Autodesk Inventor part; units mm, degrees
ref_plane "YZ Plane" through (0, 0, 0) normal (1, 0, 0) x (0, 1, 0)
ref_plane "XZ Plane" through (0, 0, 0) normal (0, 1, 0) x (-1, 0, 0)
ref_plane "XY Plane" through (0, 0, 0) normal (0, 0, 1) x (1, 0, 0)
sketch "Sketch1" plane through (0, 0, 0) normal (0, 0, 1) x (1, 0, 0)
  circle A0 centre (0, 4) radius 2 construction
  circle A1 centre (-195, 4) radius 2 construction
  circle A2 centre (195, 4) radius 2 construction
  arc A3 (213, -12) -> (215, -10) centre (213, -10) ccw construction
  line L0 (215, -10) -> (215, 10) construction
  arc A4 (215, 10) -> (213, 12) centre (213, 10) ccw construction
  line L1 (213, 12) -> (-213, 12) construction
  line L2 (94, -2.8) -> (94, -7.2) construction
  line L3 (94, -7.2) -> (87.6, -7.2) construction
  line L4 (87.6, -7.2) -> (87.6, -2.8) construction
  line L5 (87.6, -2.8) -> (94, -2.8) construction
  line L6 (-108.8, -2.8) -> (-108.8, -7.2) construction
  line L7 (-108.8, -7.2) -> (-115.2, -7.2) construction
  line L8 (-115.2, -7.2) -> (-115.2, -2.8) construction
  line L9 (-115.2, -2.8) -> (-108.8, -2.8) construction
  line L10 (115.2, -2.8) -> (115.2, -7.2) construction
  line L11 (115.2, -7.2) -> (108.8, -7.2) construction
  line L12 (108.8, -7.2) -> (108.8, -2.8) construction
  line L13 (108.8, -2.8) -> (115.2, -2.8) construction
  line L14 (-87.6, -2.8) -> (-87.6, -7.2) construction
  line L15 (-87.6, -7.2) -> (-94, -7.2) construction
  line L16 (-94, -7.2) -> (-94, -2.8) construction
  line L17 (-94, -2.8) -> (-87.6, -2.8) construction
  circle A5 centre (-101.4, -5) radius 1.6 construction
  circle A6 centre (101.4, -5) radius 1.6 construction
  line L18 (213.9083, -46) -> (-214.0917, -46) construction
  line L19 (-225, 12) -> (225, 12)
  line L20 (225, 12) -> (225, -46)
  line L21 (-225, -46) -> (-225, 12)
  line L22 (-225, -46) -> (225, -46)
  line L23 (197, -54.5741) -> (193, -54.5741)
  line L24 (2, -54.5741) -> (-2, -54.5741)
  line L25 (-195, -54.5741) -> (-197, -54.5741)
  line L26 (-108.8, -54.5741) -> (-115.2, -54.5741)
  line L27 (94, -54.5741) -> (87.6, -54.5741)
  line L28 (-225, -46) -> (225, -46)
  line L29 (225, -46) -> (225, -48)
  line L30 (225, -48) -> (-225, -48)
  line L31 (-225, -48) -> (-225, -46)
  line L32 (-195, 4) -> (-195, 0) construction
  line L33 (-197, 4) -> (-197, 0)
  line L34 (-193, 0) -> (-193, 4)
  arc A7 (-193, 4) -> (-197, 4) centre (-195, 4) ccw
  arc A8 (-197, 0) -> (-193, 0) centre (-195, 0) ccw
  line L35 (0, 4) -> (0, 0) construction
  line L36 (-2, 4) -> (-2, 0)
  line L37 (2, 0) -> (2, 4)
  arc A9 (2, 4) -> (-2, 4) centre (0, 4) ccw
  arc A10 (-2, 0) -> (2, 0) centre (0, 0) ccw
  line L38 (195, 4) -> (195, 0) construction
  line L39 (193, 4) -> (193, 0)
  line L40 (197, 0) -> (197, 4)
  arc A11 (197, 4) -> (193, 4) centre (195, 4) ccw
  arc A12 (193, 0) -> (197, 0) centre (195, 0) ccw
  circle A13 centre (0, 4) radius 2 construction
  circle A14 centre (-195, 4) radius 2 construction
  circle A15 centre (195, 4) radius 2 construction
  arc A16 (213, -12) -> (215, -10) centre (213, -10) ccw construction
  line L41 (215, -10) -> (215, 10) construction
  arc A17 (215, 10) -> (213, 12) centre (213, 10) ccw construction
  line L42 (213, 12) -> (-213, 12) construction
  arc A18 (-213, 12) -> (-215, 10) centre (-213, 10) ccw construction
  line L43 (-215, 10) -> (-215, -10) construction
  arc A19 (-215, -10) -> (-213, -12) centre (-213, -10) ccw construction
  line L44 (-213, -12) -> (213, -12) construction
  line L45 (94, -2.8) -> (94, -7.2) construction
  line L46 (94, -7.2) -> (87.6, -7.2) construction
  line L47 (87.6, -7.2) -> (87.6, -2.8) construction
  line L48 (87.6, -2.8) -> (94, -2.8) construction
  line L49 (-108.8, -2.8) -> (-108.8, -7.2) construction
  line L50 (-108.8, -7.2) -> (-115.2, -7.2) construction
  line L51 (-115.2, -7.2) -> (-115.2, -2.8) construction
  line L52 (-115.2, -2.8) -> (-108.8, -2.8) construction
  line L53 (115.2, -2.8) -> (115.2, -7.2) construction
  line L54 (115.2, -7.2) -> (108.8, -7.2) construction
  line L55 (108.8, -7.2) -> (108.8, -2.8) construction
  line L56 (108.8, -2.8) -> (115.2, -2.8) construction
  line L57 (-87.6, -2.8) -> (-87.6, -7.2) construction
  line L58 (-87.6, -7.2) -> (-94, -7.2) construction
  line L59 (-94, -7.2) -> (-94, -2.8) construction
  line L60 (-94, -2.8) -> (-87.6, -2.8) construction
  circle A20 centre (-101.4, -5) radius 1.6 construction
  circle A21 centre (101.4, -5) radius 1.6 construction
  point P0 (-213, -12)
  point P1 (-195, 2)
  point P2 (0, 2)
  point P3 (195, 2)
  dimension "d0" = 2
  dimension "d1" = 58
  dimension "d5" = 4
  dimension "d6" = 4
  dimension "d7" = 4
  dimension "d17" = 10
  dimension "d18" = 10
extrude "Extrusion2" add sketch "Sketch1" along normal blind 1
fillet "Fillet2" radius 2 4 edges at (-225, -48, 0.5) (-225, 12, 0.5) (225, 12, 0.5) (225, -48, 0.5)
sketch "Sketch2" plane through (0, 0, 1) normal (0, 0, 1) x (1, 0, 0)
  circle A0 centre (-101.4, -5) radius 1.6
  circle A1 centre (101.4, -5) radius 1.6
  line L0 (115, -3) -> (115, -7)
  line L1 (87.6, -7.2) -> (87.6, -2.8)
  line L2 (-87.8, -3) -> (-87.8, -7)
  line L3 (-115, -3) -> (-115, -7)
  line L4 (-101.4, 24.0788) -> (-101.4, -5) construction
  line L5 (-118.4, 24.0788) -> (-118.4, -5)
  line L6 (-84.4, -5) -> (-84.4, 24.0788)
  arc A2 (-84.4, 24.0788) -> (-118.4, 24.0788) centre (-101.4, 24.0788) ccw
  arc A3 (-118.4, -5) -> (-84.4, -5) centre (-101.4, -5) ccw
  line L7 (101.4, 38.8521) -> (101.4, -5) construction
  line L8 (84.4, 38.8521) -> (84.4, -5)
  line L9 (118.4, -5) -> (118.4, 38.8521)
  arc A4 (118.4, 38.8521) -> (84.4, 38.8521) centre (101.4, 38.8521) ccw
  arc A5 (84.4, -5) -> (118.4, -5) centre (101.4, -5) ccw
  point P0 (-101.4, 9.5394)
  point P1 (101.4, 16.926)
  dimension "d13" = 17
extrude "Extrusion3" cut sketch "Sketch2" against normal blind 1 contours A0 | A1 | A2 L6 A3 L5 | A4 L9 A5 L8
fillet "Fillet3" radius 2 4 edges at (-118.4, 12, 0.5) (-84.4, 12, 0.5) (84.4, 12, 0.5) (118.4, 12, 0.5)
properties part number "wiper 2"
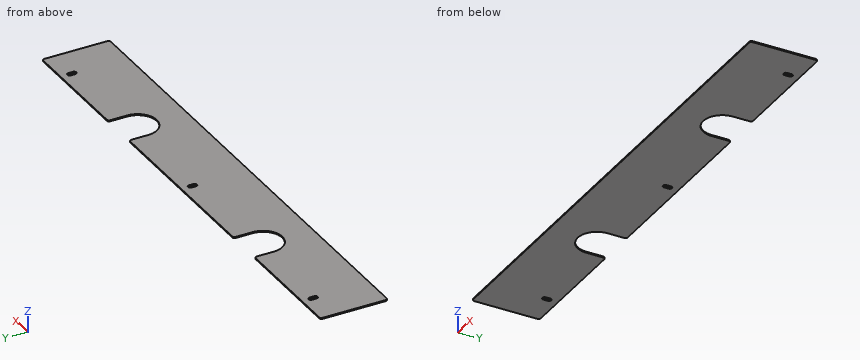
The listing builds one solid part. Answer for the finished solid, in the listing's coordinates (mm). Give positions to 0.01 mm unless a question says otherwise; leave off trailing zeros. Order: outer loops, then holes, each group sorted by start corner. A loop starts at its lowest first (then second) coordinate and runs counter-clockwise, first axis right, second up. Notation, with made-up numbers: (64, -27) -> (110, -27) arc R24 ccw to (110, -12) -> close; hole circle Ø10 at (-8.5, 83.5). An arc over 180 degrees is marked (long way). Answer as CSV lines item,"result". Start each with the question number.
Q1. Find the intervals of material crossed by L1, parallel to X at y = 6.5, z = 0.5; L2, parallel to X at y = -13, z = 0.95; L3, parallel to X at y = 2, z = 0.4, in increasing order.
Q2. A cutting plane is placed at B-B (x = 101.4). Determine the outline of the cut face in (y, z), then the cut area to 3 significant figures.
Q3. A cutting plane is placed at A-A (z = 0.35). Count the separate pieces of the cut face and the enclosed holes in it, then the cut area to 3 significant figures.
Results found:
1,L1,"-225 to -118.4, -84.4 to 84.4, 118.4 to 225"
1,L2,"-225 to -116.4, -86.4 to 86.4, 116.4 to 225"
1,L3,"-225 to -197, -193 to -118.4, -84.4 to -2, 2 to 84.4, 118.4 to 193, 197 to 225"
2,outline,"(-48, 0) -> (-22, 0) -> (-22, 1) -> (-48, 1) -> close"
2,area,"26.0 mm2"
3,separate pieces,"1"
3,enclosed holes,"3"
3,area,"24,800 mm2"
